Part model, mm, in its own coordinate system. A direction names the side the tool comes from. Round coordinates to 2 decimals unless told otherwise and drop trailing zeros. Order: outer loops, then holes, each group sorted by start corner. A loop starts at its lowest first (then second) coordinate and runs counter-clockwise, first axis right, second up. Notation, with made-up numbers: (-23, -24.5) -> (3, -24.5) arc R23 ccw to (3, -14.5) -> close; hole circle Ø5 at (-27.5, -27). An arc over 180 degrees is marked (long way). Answer as a JSON object with one key per item and string values. Group by question number.
```python
from build123d import *


with BuildPart() as f1:
    # F0 (on Front) → F1 (revolve)
    with BuildSketch(Plane.XZ):
        with BuildLine():
            add(Edge.make_bspline(
                [(8.255, 0), (8.2216796153, 2.3076537954), (8.8350885951, 8.5271520648), (12.1501012783, 16.3709643576), (17.4859554214, 20.2662519854), (19.6571610868, 19.3162634969)],
                knots=[0, 0, 0, 0, 0.3357963175, 0.6868837016, 1, 1, 1, 1], degree=3))
            Line((8.255, 0), (27.7114, 0))
            Line((27.7114, 0), (27.7114, 6.985))
            Line((27.7114, 6.985), (29.4894, 6.985))
            Line((29.4894, 6.985), (29.4894, 0))
            Line((29.4894, 0), (31.3944, 0))
            Line((31.3944, 0), (31.3944, 8.89))
            Line((31.3944, 8.89), (18.3997968841, 8.89))
            Line((18.3997968841, 8.89), (20.9748614579, 17.1817578375))
            ThreePointArc((20.9748614579, 17.1817578375), (20.7383933614, 18.509760988), (19.6571610868, 19.3162634969))
        make_face()
    revolve(axis=Axis((0, 0, 8.4439804778), (0, 0, 1)))


solid = f1.part
```
Q1. Drop flat-ended pins along their axis: pin 1 Ø2 at (x, z) = (-22, 6) entering from +Y; pin 2 Ø12 at (x, y) = (6.5, 9) entering from +Z; pin 3 Ø1 at (y, z) = (-2, 8.5) entering from -X. Give the stop position or say it passes through.
Q2. Two-plate mould, pull along Y, no slides. Class faces 4 (the cylindrical face through (-6.01, -27.05, 3.54)), 5 (the conical face through (-4.02, -18.12, 9.41)), 6 (the flat face through (7, -6, 0)): +Y half, -Y half, draft (parallel to the pull), parting line (faces both ways), or undercut.
Q3. Band-saw the part on B-B (y = 23). List the corners of the cut face in (x, z) (3 decimals).
Q4. Band-saw the part on C-C (z = 3). Count the separate pieces of the cut face and the enclosed holes in it, plus the area to 3 significant figures.
Q5. Wall check: line 1 (X direction, y = 11.5, z = 1.5); line 2 (X direction, y = -5, z = 1); line 3 (X direction, y = 25, z = 4.75). Give the ranges that are in metal, low to high. Write a range as [from, to].
Q6. Which spindle directions (+Z, -Z, +X, -X, +Y, -Y) get a long thin tool onto all of the face, cutting with end or side? Do faces 1 (the flat face through (14, -14, 8.89)), 2 (the cylindrical face through (28.128, 8.858, 3.444)), 3 (the cylindrical face through (29.945, 9.43, 4.507)). Say none if no direction does.
Q7. Band-saw the part on A-A (x = -23.5). List the corners of the cut face in (y, z) (3 decimals).
Completed:
{
 "1": {"pin 1": "y = 23.34", "pin 2": "z = 19.33", "pin 3": "x = -31.36"},
 "2": {"face 4": "undercut", "face 5": "parting line", "face 6": "draft"},
 "3": {"outline": "(-21.368, 0) -> (-18.456, 0) -> (-18.456, 6.985) -> (-15.457, 6.985) -> (-15.457, 0) -> (15.457, 0) -> (15.457, 6.985) -> (18.456, 6.985) -> (18.456, 0) -> (21.368, 0) -> (21.368, 8.89) -> (-21.368, 8.89) -> close"},
 "4": {"separate pieces": "2", "enclosed holes": "2", "area": "2,560 mm2"},
 "5": {"line 1": "[-29.21, -27.15], [-25.21, 25.21], [27.15, 29.21]", "line 2": "[-30.99, -29.06], [-27.26, -6.58], [6.58, 27.26], [29.06, 30.99]", "line 3": "[-18.99, -15.64], [-11.95, 11.95], [15.64, 18.99]"},
 "6": {"face 1": "none", "face 2": "-Z", "face 3": "+Z, -Z"},
 "7": {"outline": "(-20.817, 0) -> (-17.815, 0) -> (-17.815, 6.985) -> (-14.686, 6.985) -> (-14.686, 0) -> (14.686, 0) -> (14.686, 6.985) -> (17.815, 6.985) -> (17.815, 0) -> (20.817, 0) -> (20.817, 8.89) -> (-20.817, 8.89) -> close"}
}
